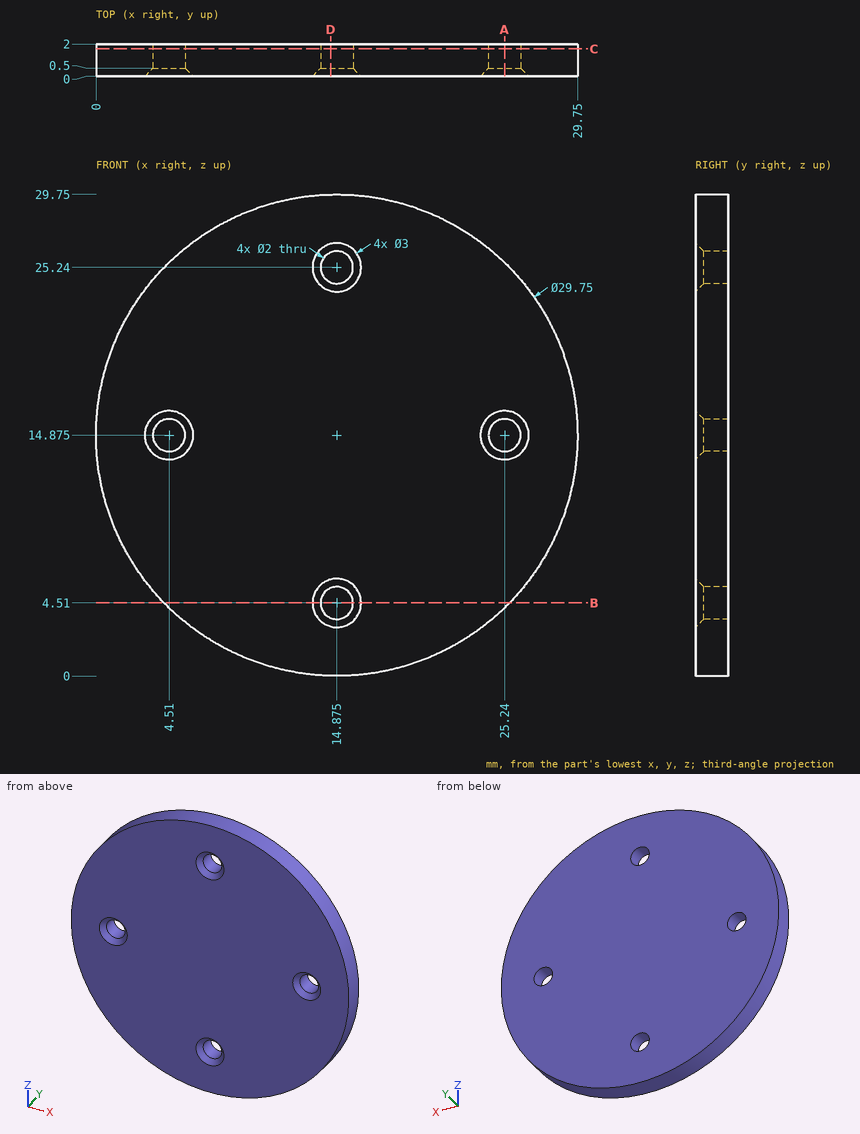
Can you work these out from the drawing? Everything is in mm from the part's minimum corner. Give positions to 0.01 mm unless a question says otherwise; leave off trailing zeros. Order: outer loops, then holes, each group sorted by start corner. A loop starts at its lowest first (then second) coordinate and runs counter-clockwise, first axis right, second up. Notation, with made-up numbers: (32.25, 6) -> (76.25, 6) arc R7 ccw to (76.25, 10) -> close; hole circle Ø2 at (81.5, 82). An arc over 180 degrees is marked (long way). Return JSON: item names as keys, results as strings.
1. Imagine slicing it at A-A on x = 25.24. List the corners of the cut face in (y, z) for me (3 decimals), then the cut area to 3 significant figures.
Answer list:
{"outline": "(0, 4.206) -> (2, 4.206) -> (2, 13.875) -> (0.5, 13.875) -> (0, 13.375) -> close; (0, 16.375) -> (0.5, 15.875) -> (2, 15.875) -> (2, 25.544) -> (0, 25.544) -> close", "area": "38.4 mm2"}
2. For pin 1 Ø1.8 at (x, z) = (14.875, 25.24) entering from -Y; pin 2 Ø1 at (x, y) = (22, 1) entering from +Z, each with a flat end and sliding along its axis, tell me the tip position at first contact or that it passes through.
Answer list:
{"pin 1": "passes through", "pin 2": "stops at z = 28.19"}
3. Imagine slicing it at B-B on z = 4.51. List the corners of the cut face in (x, y) for me (3 decimals).
Answer list:
{"outline": "(4.206, 0) -> (13.375, 0) -> (13.875, 0.5) -> (13.875, 2) -> (4.206, 2) -> close; (15.875, 0.5) -> (16.375, 0) -> (25.544, 0) -> (25.544, 2) -> (15.875, 2) -> close"}
4. Imagine slicing it at D-D on x = 14.5. Give the number of separate pieces and of enclosed holes in the cut face, then the cut area to 3 significant figures.
Answer list:
{"separate pieces": "3", "enclosed holes": "0", "area": "51.5 mm2"}
5. Imagine slicing it at C-C on y = 1.7. List the corners of the cut face in (x, z) for me (3 decimals).
Answer list:
{"outline": "circle Ø29.75 at (14.875, 14.875); hole circle Ø2 at (4.51, 14.875); hole circle Ø2 at (14.875, 4.51); hole circle Ø2 at (14.875, 25.24); hole circle Ø2 at (25.24, 14.875)"}
6. I need wall thicknesses on line 1 (X direction, y = 0.45, z = 14); line 2 (Z direction, x = 4.51, y = 1.35) (3 decimals); line 3 (X direction, y = 0.9, z = 24.75). Which ranges of each line are inside material? Lowest first, please. Write a range as from..to.
Answer list:
{"line 1": "x = 0.03..3.93, 5.09..24.66, 25.82..29.72", "line 2": "z = 4.206..13.875, 15.875..25.544", "line 3": "x = 3.75..14, 15.75..26"}
